Design review of the part shown in the three views and the two pictorial views. Dimensions are in mm from the part's minimum x, y and z. Give positions to 0.01 mm unless a question says otherwise; leave off trailing zeros. Order: outer loops, then holes, each group sorted by start corner. A loop starts at its lowest first (then second) coordinate and runs counter-clockwise, first axis right, second up. Notation, with made-up numbers: (30.25, 18) - (54.25, 18) arc R7 cw to (54.25, 26) - close; hole circle Ø3 at (50.5, 80.5). An arc over 180 degrees is marked (long way). Put each result on its own line as item: value. Start each with the question number.
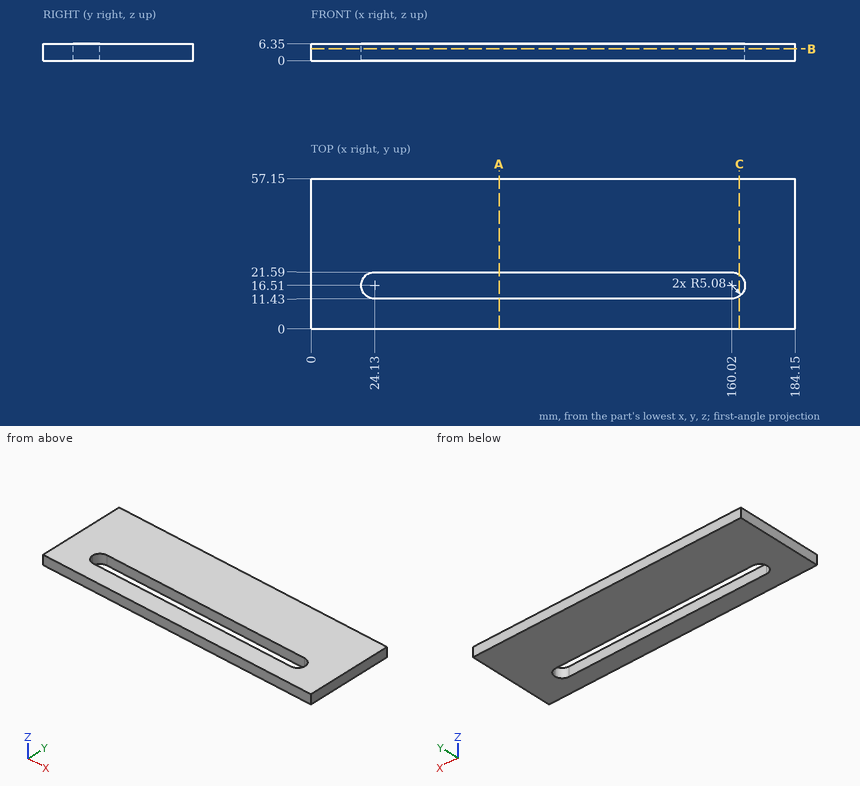
1. Clearance check with a flat-ended pin moving along its axis: pin 1 (2 mm diameter, centred on y = 16.5, z = 5, fed in from -X). State where the tip first meets the part, or that it passes through.
2. Add section B-B, the plane z = 4.5. Give the boundary of the cut face in (x, y).
3. Wall thickness on line 1 (Y direction, x = 59, z = 1); line 2 (X direction, y = 15, z = 1); line 3 (X direction, y = 19, z = 1.75): over which ranges is each line inside the solid? List them lowest first. Write a range as from..to.
4. Add section C-C, the plane x = 163. Give the boundary of the cut face in (y, z).
5. Add section A-A, the plane x = 71.5. Give the boundary of the cut face in (y, z).
Found:
1. pin 1: stops at x = 0
2. outline: (0, 0) - (184.15, 0) - (184.15, 57.15) - (0, 57.15) - close; hole (19.05, 16.51) arc R5.08 ccw to (24.13, 11.43) - (160.02, 11.43) arc R5.08 ccw to (165.1, 16.51) arc R5.08 ccw to (160.02, 21.59) - (24.13, 21.59) arc R5.08 ccw to start
3. line 1: y = 0..11.43, 21.59..57.15
3. line 2: x = 0..19.28, 164.87..184.15
3. line 3: x = 0..19.7, 164.45..184.15
4. outline: (0, 0) - (12.4, 0) - (12.4, 6.35) - (0, 6.35) - close; (20.62, 0) - (57.15, 0) - (57.15, 6.35) - (20.62, 6.35) - close
5. outline: (0, 0) - (11.43, 0) - (11.43, 6.35) - (0, 6.35) - close; (21.59, 0) - (57.15, 0) - (57.15, 6.35) - (21.59, 6.35) - close
